Autodesk Inventor part; units mm, degrees
sketch "Sketch1" plane through (0, 0, 0) normal (0, 0, 1) x (1, 0, 0)
  line L0 (0, 2.8582) -> (0, -2.8582) construction
  line L1 (-5.7775, 0) -> (5.7775, 0) construction
  line L2 (0, 0) -> (4, 0)
  line L3 (4, 0) -> (-4, 0)
  circle A0 centre (0, 0) radius 4
  line L4 (0, 0) -> (-2, 3.4641)
  line L5 (0, 0) -> (4, 0) construction
  line L6 (0, 0) -> (2, 3.4641)
  line L7 (0, 0) -> (4, 0) construction
  line L8 (0, 0) -> (4, 0)
  line L9 (0, 0) -> (2, -3.4641)
  line L10 (0, 0) -> (-2, -3.4641)
  line L11 (-2, 3.4641) -> (2, 3.4641)
  line L12 (2, 3.4641) -> (4, 0)
  line L13 (4, 0) -> (2, -3.4641)
  line L14 (2, -3.4641) -> (-2, -3.4641)
  line L15 (-2, -3.4641) -> (-4, 0)
  line L16 (-4, 0) -> (-2, 3.4641)
  dimension "d1" = 4
  dimension "d2" = 8
  dimension "d3" = 120
  dimension "d4" = 60
extrude "Extrusion1" add sketch "Sketch1" along normal blind 43.5 contours L6 L12 L2 | L10 L15 L3 | L3 L16 L4 | L4 L11 L6 | L2 L13 L9 | L9 L14 L10
sketch "Sketch5" plane through (0, 0, 43.5) normal (0, 0, 1) x (1, 0, 0)
  point P0 (0, 0)
  point P1 (0, 0)
hole "Hole2" at (0, 0, 43.5) direction (0, 0, -1) diameter 3.4587 depth 8
sketch "Sketch6" plane through (0, 0, 0) normal (0, 0, -1) x (-1, 0, 0)
  point P0 (0, 0)
  point P1 (0, 0)
hole "Hole3" at (0, 0, 0) direction (0, 0, 1) diameter 3.4587 depth 10.8
ref_plane "Work Plane1" through (0, 0, 5.4) normal (0, 0, -1) x (-1, 0, 0)
properties part number "Steun stuk" material "S235"
Source: CAD feature listing. Evaluate the final solid. Frame: model axes, mm. A direction names the side the tool comes from. Coordinates: 2 decimals unless noted, no trailing zeros. Order: outer loops, then holes, each group sorted by start corner. A loop starts at its lowest first (then second) coordinate and runs counter-clockwise, first axis right, second up. Notation, with made-up numbers: M 3.5,35 L 20.5,35 A25 cw 20.5,65 Z; hole C 58.5,-34.75 d7. An arc over 180 degrees is marked long. Write each question's results on one line, items separated by ' | '. Start each with the question number.
Item 1: First-contact query: pin 1 Ø3 at (y, z) = (-2, 23) entering from +X; pin 2 Ø1.7 at (x, y) = (-0.5, -0.5) entering from -Z. Flat tips, straight axial feed; report the tip coordinate or a pass-through.
Item 2: Cut plane C-C (z = 25.5). Return loops of the section in (x, y), and give its area (3 significant figures).
Item 3: Cut plane D-D (y = -0.75). Return loops of the section in (x, z).
Item 4: Draft query along X for faces 1 (the face through (1, 2, 43.5)), 2 (the face through (-2.986, -1.756, 21.446)), 3 (the face through (-0.52, -1.65, 39.44)). Return one class per face: pulls with the +X half, pulls with the -X half, needs draft (parallel to the pull), parting line crosses it, or undercut.
Item 5: Cut plane A-A (z = 6). Return loops of the section in (x, y).
Item 6: Set-up query: faces 4 (the face through (0, 0, 35.5)), 5 (the face through (1, 2, 0)), 6 (the face through (0, 0, 10.8)). Return all of +Z, -Z, +X, -X, +Y, -Y with unobstructed straight access to the full face (end or side cutting, diameter ignored); none if empty.
Item 7: Line query: probe 1 along X at (y, z) = (0, 8.25); probe 2 along Y at (x, z) = (0, 38); probe 3 along Z at (x, y) = (1, -1). Output: solid intervals per line, ascending.
Item 8: Cut plane B-B (x = 0). Return loops of the section in (y, z).
Checked values:
1) pin 1: stops at x = 3.71 | pin 2: stops at z = 10.8
2) outline: M -4,0 L -2,-3.46 L 2,-3.46 L 4,0 L 2,3.46 L -2,3.46 Z | area: 41.6 mm2
3) outline: M -3.57,0 L -1.56,0 L -1.56,10.8 L 1.56,10.8 L 1.56,0 L 3.57,0 L 3.57,43.5 L 1.56,43.5 L 1.56,35.5 L -1.56,35.5 L -1.56,43.5 L -3.57,43.5 Z
4) face 1: needs draft | face 2: pulls with the -X half | face 3: undercut
5) outline: M -4,0 L -2,-3.46 L 2,-3.46 L 4,0 L 2,3.46 L -2,3.46 Z; hole C 0,0 d3.46
6) face 4: +Z | face 5: -Z, +X, -X, +Y, -Y | face 6: -Z
7) probe 1: x = -4 to -1.73, 1.73 to 4 | probe 2: y = -3.46 to -1.73, 1.73 to 3.46 | probe 3: z = 10.8 to 35.5
8) outline: M -3.46,0 L -1.73,0 L -1.73,10.8 L 1.73,10.8 L 1.73,0 L 3.46,0 L 3.46,43.5 L 1.73,43.5 L 1.73,35.5 L -1.73,35.5 L -1.73,43.5 L -3.46,43.5 Z
